```python
from build123d import *
from build123d.topology import SkipClean

# Parameters (mm, degrees)
UPPER_DEPTH         = 1.5
LOWER_DEPTH         = 1.5
BOSS_EXTRUDE1_DEPTH = 12.7
SKETCH3_R           = 2.159
CUT_EXTRUDE3_DEPTH  = 25.4
SKETCH21_R          = 14.2875
CUT_EXTRUDE28_DEPTH = 874.615346647
SKETCH8_R           = 12.7
CUT_EXTRUDE9_DEPTH  = 909.841508723
SKETCH7_R           = 14.2875
CUT_EXTRUDE10_DEPTH = 768.787550437
SKETCH6_R           = 14.2875
CUT_EXTRUDE11_DEPTH = 805.372191991
CUT_EXTRUDE13_DEPTH = 5.08
CUT_EXTRUDE16_DEPTH = 2.54
CUT_EXTRUDE22_DEPTH = 2.54
SKETCH20_R          = 2.159
CUT_EXTRUDE25_DEPTH = 5.08
SKETCH19_R          = 2.159
CUT_EXTRUDE26_DEPTH = 5.08
SKETCH18_R          = 2.159
CUT_EXTRUDE27_DEPTH = 5.08
SKETCH23_R          = 2.159
CUT_EXTRUDE29_DEPTH = 755.225962057
SKETCH24_W          = 4.7625
SKETCH24_H          = 406.4
BOSS_EXTRUDE2_DEPTH = 19.05


# Read off the part's stored shape, not the designer's step: Mirror1
with BuildPart() as part:
    # Sketch1 → Upper (new body)
    with BuildSketch(Plane.XY):
        Polygon((-268.322950018, 0), (268.322950018, 0), (291.817849942, -95.25), (-291.817849942, -95.25), align=None)
    extrude(amount=UPPER_DEPTH)

    # Sketch2 → Lower (add)
    with BuildSketch(Plane(origin=(0, -47.82449055, -47.624582187), x_dir=(1, 0, 0), z_dir=(0, 0.7085861902250874, 0.7056242704317195))):
        Polygon((-292.843249974, -408.979811759), (-213.216599982, -684.467611759), (-211.306786287, -681.927611759), (-290.367685881, -408.397163128), (-314.93135919, -274.122656346), (-289.573528128, -69.750711759), (-291.817849942, -67.210711759), (-317.5, -274.196511759), align=None)
        Polygon((-213.216599982, -684.467611759), (-211.306786287, -681.927611759), (-290.367685881, -408.397163128), (-314.93135919, -274.122656346), (-289.573528128, -69.750711759), (-291.817849942, -67.210711759), (291.817849942, -67.210711759), (289.573528128, -69.750711759), (314.93135919, -274.122656346), (290.367685881, -408.397163128), (211.306786287, -681.927611759), (213.216599982, -684.467611759), align=None)
        Polygon((213.216599982, -684.467611759), (211.306786287, -681.927611759), (290.367685881, -408.397163128), (314.93135919, -274.122656346), (289.573528128, -69.750711759), (291.817849942, -67.210711759), (317.5, -274.196511759), (292.843249974, -408.979811759), align=None)
    extrude(amount=LOWER_DEPTH)

    # Sketch2<3> → Boss-Extrude1 (add)
    with BuildSketch(Plane(origin=(0, -47.82449055, -47.624582187), x_dir=(1, 0, 0), z_dir=(0, 0.7085861902250874, 0.7056242704317195))):
        Polygon((213.216599982, -684.467611759), (211.306786287, -681.927611759), (290.367685881, -408.397163128), (314.93135919, -274.122656346), (289.573528128, -69.750711759), (291.817849942, -67.210711759), (317.5, -274.196511759), (292.843249974, -408.979811759), align=None)
    extrude(amount=-BOSS_EXTRUDE1_DEPTH)

    # Sketch3 → Cut-Extrude3 (cut)
    with BuildSketch(Plane(origin=(0, 0, 0), x_dir=(-1, 0, 0), z_dir=(0, 0, -1))):
        with Locations((-241.3, -5.08)):
            Circle(SKETCH3_R)
        with Locations((0, -5.08)):
            Circle(SKETCH3_R)
        with Locations((241.3, -5.08)):
            Circle(SKETCH3_R)
    extrude(amount=-CUT_EXTRUDE3_DEPTH, mode=Mode.SUBTRACT)

    # Sketch21 → Cut-Extrude28 (cut, through all)
    with BuildSketch(Plane(origin=(196.85, -539.746170446, 446.36474374), x_dir=(-0.9557127001633002, 0.25055659462572005, -0.15438467422686922), z_dir=(-0.29430126528197925, -0.8136564393089987, 0.5013481465253741))):
        with BuildLine():
            ThreePointArc((0, -14.2875), (-14.2875, 0), (0, 14.2875))
            Line((0, 14.2875), (-38.1, 14.2875))
            Line((-38.1, 14.2875), (-38.1, -14.2875))
            Line((-38.1, -14.2875), (0, -14.2875))
        make_face()
        Circle(SKETCH21_R)
    extrude(amount=-CUT_EXTRUDE28_DEPTH, mode=Mode.SUBTRACT)

    # Sketch8 → Cut-Extrude9 (cut, through all)
    with BuildSketch(Plane(origin=(255.6256, 12.775047317, 0.0545235), x_dir=(0.9817895969366798, 0.189921913110119, 0.004342150101546657), z_dir=(-0.18997154351879111, 0.9815331026321988, 0.022440612520550327))):
        Circle(SKETCH8_R)
        with BuildLine():
            ThreePointArc((12.7, 0), (8.980256121, -8.980256121), (0, -12.7))
            Line((0, -12.7), (50.8, -12.7))
            Line((50.8, -12.7), (50.8, 12.7))
            Line((50.8, 12.7), (0, 12.7))
            ThreePointArc((0, 12.7), (8.980256121, 8.980256121), (12.7, 0))
        make_face()
    extrude(amount=-CUT_EXTRUDE9_DEPTH, mode=Mode.SUBTRACT)

    # Sketch7 → Cut-Extrude10 (cut, symmetric)
    with BuildSketch(Plane(origin=(0, 0, -5.754260468), x_dir=(-1, 0, 0), z_dir=(0, 0, -1))):
        with Locations((-304.8, -241.296170446)):
            Circle(SKETCH7_R)
        with BuildLine():
            Line((-355.6, -255.583670446), (-304.8, -255.583670446))
            ThreePointArc((-304.8, -255.583670446), (-319.0875, -241.296170446), (-304.8, -227.008670446))
            Line((-304.8, -227.008670446), (-355.6, -227.008670446))
            Line((-355.6, -227.008670446), (-355.6, -255.583670446))
        make_face()
    extrude(amount=CUT_EXTRUDE10_DEPTH, both=True, mode=Mode.SUBTRACT)

    # Sketch6 → Cut-Extrude11 (cut, through all)
    with BuildSketch(Plane(origin=(228.6, -539.746170446, 198.722727079), x_dir=(0.9702139044987836, -0.23690600809094062, -0.050601609140820056), z_dir=(0.2422498287248624, 0.948811829172378, 0.202660142369784))):
        Circle(SKETCH6_R)
        with BuildLine():
            ThreePointArc((14.2875, 0), (10.102788136, -10.102788136), (0, -14.2875))
            Line((0, -14.2875), (50.8, -14.2875))
            Line((50.8, -14.2875), (50.8, 14.2875))
            Line((50.8, 14.2875), (0, 14.2875))
            ThreePointArc((0, 14.2875), (10.102788136, 10.102788136), (14.2875, 0))
        make_face()
    extrude(amount=CUT_EXTRUDE11_DEPTH, mode=Mode.SUBTRACT)

    # Sketch12 → Cut-Extrude13 (cut)
    with BuildSketch(Plane(origin=(279.180551252, 24.44271802, -24.545318473), x_dir=(-0.0869176220205297, -0.007609781256081438, -0.9961864374762041), z_dir=(0.9923902182248356, 0.08688540143887281, -0.0872501105355694))):
        with BuildLine():
            ThreePointArc((-34.458545921, -142.642226363), (-35.363095323, -147.648027336), (-38.159492817, -151.897311282))
            Line((-38.159492817, -151.897311282), (-34.334674949, -148.059274691))
            Line((-34.334674949, -148.059274691), (-34.458545921, -142.642226363))
        make_face()
        with BuildLine():
            ThreePointArc((-135.708080175, -249.783030443), (-139.788854201, -252.528666144), (-144.606803116, -253.517908429))
            Line((-144.606803116, -253.517908429), (-139.390384316, -253.478060774))
            Line((-139.390384316, -253.478060774), (-135.708080175, -249.783030443))
        make_face()
        Polygon((-34.458545921, -142.642226363), (-34.334674949, -148.059274691), (-33.456000975, -142.287544019), align=None)
    extrude(amount=-CUT_EXTRUDE13_DEPTH, mode=Mode.SUBTRACT)


with BuildPart() as body_2:
    # of the pieces the cut leaves, the one that is kept (cut_extrude13_keep)
    add(part.part.solids().sort_by_distance((-268.322950018, 0, 0))[0])

    # Sketch9 → Cut-Extrude16 (cut)
    with BuildSketch(Plane(origin=(379.361144518, -77.371751981, 77.696526699), x_dir=(0.19278613597149513, -0.03931926427703094, -0.9804527021911323), z_dir=(0.9606757859804161, -0.19593247679954207, 0.19675492056390054))):
        with BuildLine():
            Line((-176.807332276, -298.778278327), (-178.232267114, -292.159968301))
            ThreePointArc((-178.232267114, -292.159968301), (-178.434275143, -298.314516716), (-181.507674694, -303.650572247))
            Line((-181.507674694, -303.650572247), (-176.807332276, -298.778278327))
        make_face()
        with BuildLine():
            Line((-331.617972049, -441.042646452), (-332.474146327, -440.216866681))
            Line((-332.474146327, -440.216866681), (-322.519098896, -449.820583633))
            Line((-322.519098896, -449.820583633), (-313.701575889, -440.680491291))
            ThreePointArc((-313.701575889, -440.680491291), (-322.58500773, -444.56037453), (-331.617972049, -441.042646452))
        make_face()
        Polygon((-322.519098896, -449.820583633), (-332.474146327, -440.216866681), (-335.674588136, -441.430740469), (-359.267836197, -484.804221539), (-357.714104356, -486.303119554), align=None)
    extrude(amount=-CUT_EXTRUDE16_DEPTH, mode=Mode.SUBTRACT)

    # Sketch10 → Cut-Extrude22 (cut)
    with BuildSketch(Plane(origin=(355.754903335, -45.922355027, 46.115118142), x_dir=(0.12646080723028635, -0.01632409850759065, -0.9918372790143446), z_dir=(0.9836757682395201, -0.12697704918987876, 0.12751004649603565))):
        with BuildLine():
            ThreePointArc((-116.91323791, -214.396901236), (-113.138471271, -223.354168193), (-116.803052388, -232.357075488))
            Line((-116.803052388, -232.357075488), (-97.690742096, -213.008809877))
            Line((-97.690742096, -213.008809877), (-117.980385141, -213.342768044))
            Line((-117.980385141, -213.342768044), (-116.91323791, -214.396901236))
        make_face()
        with BuildLine():
            ThreePointArc((-167.632633505, -283.814184614), (-176.500013499, -287.588081665), (-185.464014694, -284.04980391))
            Line((-185.464014694, -284.04980391), (-182.326299222, -298.68925428))
            Line((-182.326299222, -298.68925428), (-167.632633505, -283.814184614))
        make_face()
        with BuildLine():
            ThreePointArc((-185.464014694, -284.04980391), (-185.528633184, -283.987314925), (-185.592807757, -283.924370136))
            Line((-185.592807757, -283.924370136), (-185.898455633, -283.622449687))
            Line((-185.898455633, -283.622449687), (-186.418418258, -302.057831208))
            Line((-186.418418258, -302.057831208), (-176.55762787, -302.057831208))
            Line((-176.55762787, -302.057831208), (-167.632633505, -283.814184614))
            Line((-167.632633505, -283.814184614), (-182.326299222, -298.68925428))
            Line((-182.326299222, -298.68925428), (-185.464014694, -284.04980391))
        make_face()
    extrude(amount=-CUT_EXTRUDE22_DEPTH, mode=Mode.SUBTRACT)

    # Mirror1
    split(bisect_by=Plane(origin=(0, 0, 0), x_dir=(0, 0, 1), z_dir=(1, 0, 0)), keep=Keep.TOP)

    # Mirror1 2: body 2 across plane


with BuildPart() as body_2_1:
    with SkipClean():  # the faces are left unmerged after this step: merging them gives an invalid solid
        add(body_2.part)
        add(body_2.part.mirror(Plane(origin=(0, 0, 0), x_dir=(0, 0, 1), z_dir=(1, 0, 0))))

    # Sketch20 → Cut-Extrude25 (cut)
    with SkipClean():  # the faces are left unmerged after this step: merging them gives an invalid solid
        with BuildSketch(Plane(origin=(0, -47.82557375, -47.624577646), x_dir=(1, 0, 0), z_dir=(1.6140263867400147e-15, 0.7085942146752751, 0.7056162122065581))):
            with Locations(Location((0, -679.386829065, 0), (0, 0, 269.999999992))):
                Circle(SKETCH20_R)
        cut_extrude25 = extrude(amount=CUT_EXTRUDE25_DEPTH, mode=Mode.SUBTRACT)

    # Sketch19 → Cut-Extrude26 (cut)
    with SkipClean():  # the faces are left unmerged after this step: merging them gives an invalid solid
        with BuildSketch(Plane(origin=(0, -47.82557375, -47.624577646), x_dir=(1, 0, 0), z_dir=(1.6417819623556435e-15, 0.7085942146752751, 0.7056162122065581))):
            with Locations(Location((-260.942318198, -408.979044635, 0), (0, 0, 269.999999991))):
                Circle(SKETCH19_R)
        cut_extrude26 = extrude(amount=CUT_EXTRUDE26_DEPTH, mode=Mode.SUBTRACT)

    # Sketch18 → Cut-Extrude27 (cut)
    with SkipClean():  # the faces are left unmerged after this step: merging them gives an invalid solid
        with BuildSketch(Plane(origin=(0, -47.82557375, -47.624577646), x_dir=(1, 0, 0), z_dir=(1.6972931135869015e-15, 0.7085942146752751, 0.7056162122065581))):
            with Locations(Location((-287.02, -274.195777815, 0), (0, 0, 269.999999991))):
                Circle(SKETCH18_R)
        cut_extrude27 = extrude(amount=CUT_EXTRUDE27_DEPTH, mode=Mode.SUBTRACT)

    # Sketch23 → Cut-Extrude29 (cut, symmetric)
    with SkipClean():  # the faces are left unmerged after this step: merging them gives an invalid solid
        with BuildSketch(Plane(origin=(0, -47.82557375, -47.624577646), x_dir=(1, 0, 0), z_dir=(1.7528042648181593e-15, 0.708594214675275, 0.7056162122065582))):
            with Locations(Location((-185.162281701, -679.386829065, 0), (0, 0, 269.999999991))):
                Circle(SKETCH23_R)
        cut_extrude29 = extrude(amount=CUT_EXTRUDE29_DEPTH, both=True, mode=Mode.SUBTRACT)

    # Mirror2: Cut-Extrude25, Cut-Extrude26, Cut-Extrude27, Cut-Extrude29 across plane
    with SkipClean():  # the faces are left unmerged after this step: merging them gives an invalid solid
        add(cut_extrude25.mirror(Plane(origin=(0, 0, 0), x_dir=(0, 0, 1), z_dir=(1, 0, 0))), mode=Mode.SUBTRACT)
        add(cut_extrude26.mirror(Plane(origin=(0, 0, 0), x_dir=(0, 0, 1), z_dir=(1, 0, 0))), mode=Mode.SUBTRACT)
        add(cut_extrude27.mirror(Plane(origin=(0, 0, 0), x_dir=(0, 0, 1), z_dir=(1, 0, 0))), mode=Mode.SUBTRACT)
        add(cut_extrude29.mirror(Plane(origin=(0, 0, 0), x_dir=(0, 0, 1), z_dir=(1, 0, 0))), mode=Mode.SUBTRACT)

    # Sketch24 → Boss-Extrude2 (add)
    with SkipClean():  # the faces are left unmerged after this step: merging them gives an invalid solid
        with BuildSketch(Plane(origin=(0, -47.82449055, -47.624582187), x_dir=(1, 0, 0), z_dir=(0, -0.7085861902250873, -0.7056242704317196))):
            with Locations((0, 270.410711759)):
                Rectangle(SKETCH24_W, SKETCH24_H)
        extrude(amount=BOSS_EXTRUDE2_DEPTH)


solid = body_2_1.part
```
For this review, take the finished solid that the model builds, in its own axes (mm). A direction names the side the tool comes from. Round coordinates to 2 decimals unless told otherwise and drop trailing zeros. Order: outer loops, then holes, each group sorted by start corner. A loop starts at its lowest first (then second) coordinate and runs counter-clockwise, first axis right, second up. Notation, with made-up numbers: (-22.5, 82) -> (7.5, 82) arc R27 ccw to (7.5, 99) -> close; hole circle Ø3 at (55, 14.5). An arc over 180 degrees is marked (long way). Use a Markdown table: item, result.
Item 1: Take a section at B-B (z = 72). State the section outline as (x, y) points, plus the area to 3 significant figures.
Resolved:
| item | result |
|---|---|
| outline | (-305.99, -184.87) -> (-303.44, -184.87) -> (-301.87, -166.95) -> (-2.38, -166.95) -> (-2.38, -193.83) -> (2.38, -193.83) -> (2.38, -166.95) -> (301.87, -166.95) -> (303.44, -184.87) -> (305.99, -184.87) -> (304.24, -164.83) -> (-304.24, -164.83) -> close |
| area | 1,510 mm² |
Item 2: Machinability: for faces 4 (the cylindrical face through (-201.048, -505.937, 413.098)), 5 (the flat face through (2.381, -243, 135)), 6 (the flat face through (-301.873, -171.427, 67.623)), 7 (the flat face through (302.108, -295.153, 191.868)), which of the approach directions +Z, -Z, +X, -X, +Y, -Y give a long, thin tool a straight path to every point of the face, cutting with its end or side? Answer none if there is none.
Resolved:
| item | result |
|---|---|
| face 4 | +Z, -X |
| face 5 | -Z, -Y |
| face 6 | -Y |
| face 7 | -Z |
Item 3: Draft analysis for pull direction Y (two halves, no side actions). For faces 1 (the flat face through (254.649, -427.636, 324.908)), 2 (the flat face through (4.412, -309.137, 216.911)), 3 (the flat face through (-2.381, -243, 135)), state which applies: +Y half, -Y half, draft (parallel to the pull), parting line (faces both ways), or undercut.
Resolved:
| item | result |
|---|---|
| face 1 | undercut |
| face 2 | +Y half |
| face 3 | draft |
Item 4: Take a section at D-D (z = 349). State the section outline as (x, y) points.
Resolved:
| item | result |
|---|---|
| outline | (-249.7, -440.67) -> (-245.61, -460.71) -> (-242.97, -460.71) -> (-246.62, -442.79) -> (246.62, -442.79) -> (242.97, -460.71) -> (245.61, -460.71) -> (249.7, -440.67) -> close |
Item 5: Take a section at C-C (x = 147.5). State the section outline as (y, z) points, plus the area to 3 significant figures.
Resolved:
| item | result |
|---|---|
| outline | (-530.8, 437.38) -> (-95.25, 0) -> (0, 0) -> (0, 1.5) -> (-94.63, 1.5) -> (-529.74, 438.44) -> close |
| area | 1,070 mm² |
Item 6: Take a section at A-A (y = -169). State the section outline as (x, z) points.
Resolved:
| item | result |
|---|---|
| outline | (-304.97, 76.19) -> (-303.2, 56.06) -> (-300.64, 56.06) -> (-302.23, 74.06) -> (-2.38, 74.06) -> (-2.38, 47.06) -> (2.38, 47.06) -> (2.38, 74.06) -> (302.23, 74.06) -> (300.64, 56.06) -> (303.2, 56.06) -> (304.97, 76.19) -> close |
Item 7: For line 1 along Y through (x, z) = (0, 0.85); line 2 along Z through (x, y) = (13.5, -85.5); line 3 along X through (y, z) = (-5, 1), list the stretches that pass through material, from the lowest coordinate up. Write a range as [from, to].
Resolved:
| item | result |
|---|---|
| line 1 | y = [-122.98, -7.24], [-2.92, 0] |
| line 2 | z = [0, 1.5] |
| line 3 | x = [-246.2, -243.46], [-239.14, -2.16], [2.16, 239.14], [243.46, 246.2] |
Item 8: For pin 1 (3 mm diameter, centred on x = 312, z = 122.5, fed in from -Y); pin 2 (3 mm diameter, centred on x = -229.5, z = 322.5, fed in from -Y); pin 3 (10 mm diameter, centred on x = -158, y = -325, fed in from +Z), all flat-tipped, find the tip position at first contact; note any pin that passes through.
Resolved:
| item | result |
|---|---|
| pin 1 | stops at y = -227.01 |
| pin 2 | stops at y = -417.9 |
| pin 3 | stops at z = 237.86 |
